from build123d import *

# Parameters (mm, degrees)
F1_DEPTH = 63.5
F0_W     = 25.4
F0_H     = 4.7752
F0_H_2   = 18.7659815103
F0_H_3   = 5.0338184897
F2_DEPTH = 25.4
F3_DEPTH = 7.9375


with BuildPart() as f1:
    # F0 (on Front) → F1 (new body, symmetric)
    with BuildSketch(Plane.XZ):
        Polygon((41.275, -9.525), (41.275, 9.525), (22.225, 9.525), (-41.275, 9.525), (-41.275, -9.525), align=None)
    extrude(amount=F1_DEPTH, both=True)

    # F0 (on Front) → F2 (join, symmetric)
    with BuildSketch(Plane.XZ):
        with BuildLine():
            Line((22.225, 9.525), (41.275, 9.525))
            Line((41.275, 9.525), (41.275, 27.0002))
            ThreePointArc((41.275, 27.0002), (45.9246798487, 38.2255201513), (57.15, 42.8752))
            Line((57.15, 42.8752), (60.325, 42.8752))
            Line((60.325, 42.8752), (60.325, 61.6411815103))
            Line((60.325, 61.6411815103), (52.705, 61.6411815103))
            ThreePointArc((52.705, 61.6411815103), (30.929805016, 50.0708956982), (22.225, 27.0002))
            Line((22.225, 27.0002), (22.225, 9.525))
        make_face()
        with Locations((73.025, 40.4876)):
            Rectangle(F0_W, F0_H)
        with Locations((73.025, 52.2581907552)):
            Rectangle(F0_W, F0_H_2)
        with Locations((73.025, 64.1580907552)):
            Rectangle(F0_W, F0_H_3)
    extrude(amount=F2_DEPTH, both=True)

    # F0 (on Front) → F3 (join, symmetric)
    with BuildSketch(Plane.XZ):
        with BuildLine():
            Line((-41.275, 9.525), (22.225, 9.525))
            Line((22.225, 9.525), (22.225, 27.0002))
            ThreePointArc((22.225, 27.0002), (30.929805016, 50.0708956982), (52.705, 61.6411815103))
            add(Edge.make_bspline(
                [(-41.275, 9.525), (-26.7878733575, 47.4557615817), (10.0529832694, 61.8960684807), (52.705, 61.6411815103)],
                knots=[0, 0, 0, 0, 107.4631880004, 107.4631880004, 107.4631880004, 107.4631880004], degree=3))
        make_face()
    extrude(amount=F3_DEPTH, both=True)


solid = f1.part
Check sheet for the modelled part. Datum: model origin and axes. Units: mm. A direction names the side the tool comes from. Give positions to 0.01 mm unless a question says otherwise; leave off trailing zeros. Write each loop counter-clockwise with the first axis right and the second up, starting at its lowest first coordinate (ties: lowest second). Pieces come first, ordered by that corner, then holes. Notation, with made-up numbers: M 88,52 L 111,52 A11 ccw 111,58 Z; hole C 17,28.25 d4. An arc over 180 degrees is marked long. Use one line per item in the form item = value.
(1) Material ranges on line 1 along Y through (x, z) = (79, 42.5); line 2 along Z through (x, y) = (-34, 19.5) (3 decimals); line 3 along X through (y, z) = (-8, 25.5) (3 decimals), recorded low to high.
Answer block:
line_1 = -25.4 to 25.4
line_2 = -9.525 to 9.525
line_3 = 22.225 to 41.275
(2) Section check C-C on y = 46. Record the boundary of the cut face in (x, z) (3 decimals).
Answer block:
outline = M -41.275,-9.525 L 41.275,-9.525 L 41.275,9.525 L -41.275,9.525 Z
(3) Draft check along X on faces 5 (the flat face through (60.325, 0, 40)), 6 (the cylindrical face through (31.16, 16.55, 50.33)), 7 (the flat face through (54, -25.4, 45)). Enter one of: pulls with the +X half, pulls with the -X half, needs draft (parallel to the pull), parting line crosses it, or undercut.
Answer block:
face_5 = undercut
face_6 = pulls with the -X half
face_7 = needs draft
(4) Section check B-B on x = 74.5. Record the boundary of the cut face in (y, z) (3 decimals).
Answer block:
outline = M -25.4,38.1 L 25.4,38.1 L 25.4,66.675 L -25.4,66.675 Z
(5) Tool access check on faces 1 (the flat face through (59, 0, 42.875)), 2 (the flat face through (-5, 7.938, 30)), 3 (the flat face through (60.325, 0, 64)), 4 (the flat face through (41.275, -1, 4)). Record the directions out of +Z, -Z, +X, -X, +Y, -Y that give a thin tool (end or side, any length) a straight path to the whole face; none if there is none.
Answer block:
face_1 = -Z, +Y, -Y
face_2 = +Z, -X, +Y
face_3 = +Z, -X, +Y, -Y
face_4 = -Z, +X, +Y, -Y
(6) Depth check by flat-ended pin: P1, Ø1.5, axis at x = 42, z = 34, coming from the -Y side; P2, Ø16.5, axis at x = 11.5, y = -27, coming from the +Z side (3 decimals); P3, Ø10, axis at x = 45, z = 44, coming from the +Y side; P4, Ø8.5, axis at x = 57.5, y = 0, coming from the +Z side (3 decimals). Enter the tip coordinate at first touch or a pass-through.
Answer block:
P1 = -25.4
P2 = 9.525
P3 = 25.4
P4 = 66.675
(7) Section check A-A on y = 21. Record the boundary of the cut face in (x, z) (3 decimals).
Answer block:
outline = M -41.275,-9.525 L 41.275,-9.525 L 41.275,27 A15.875 cw 57.15,42.875 L 60.325,42.875 L 60.325,38.1 L 85.725,38.1 L 85.725,66.675 L 60.325,66.675 L 60.325,61.641 L 52.705,61.641 A34.925 ccw 22.225,27 L 22.225,9.525 L -41.275,9.525 Z
